from build123d import *

# Parameters (mm, degrees)
BOSS_EXTRU_1_DEPTH = 5
BOSS_EXTRU_2_DEPTH = 5


with BuildPart() as part:
    # Esquisse1 → Boss.-Extru.1 (new body)
    with BuildSketch(Plane(origin=(0, 0, 0), x_dir=(1, 0, 0), z_dir=(0, 1, 0))):
        with BuildLine():
            Line((-45.607160176, -54.708924596), (-20.666600132, -11.510607431))
            Line((-20.666600132, -11.510607431), (-20.260750016, -11.207654407))
            Line((-20.260750016, -11.207654407), (-0.260750016, -11.207654407))
            Line((-0.260750016, -11.207654407), (19.739249984, -11.207654407))
            Line((19.739249984, -11.207654407), (20.085660146, -11.407654407))
            Line((20.085660146, -11.407654407), (45.085660146, -54.708924596))
            Line((45.085660146, -54.708924596), (45.085660146, 5.291075404))
            ThreePointArc((45.085660146, 5.291075404), (-1.258158233, 50.543971712), (-45.394459717, 3.135522912))
            Line((-45.394459717, 3.135522912), (-45.607160176, -54.708924596))
        make_face()
    extrude(amount=BOSS_EXTRU_1_DEPTH)

    # Esquisse3 → Boss.-Extru.2 (add)
    with BuildSketch(Plane.XZ):
        with BuildLine():
            Line((-17.273069059, 14.232839193), (-17.133250941, 13.990667109))
            Line((-17.133250941, 13.990667109), (-16.960798401, 13.691970548))
            ThreePointArc((-16.960798401, 13.691970548), (-16.911924508, 13.553212004), (-16.916519184, 13.406169561))
            Line((-16.916519184, 13.406169561), (-16.926742719, 13.359617338))
            ThreePointArc((-16.926742719, 13.359617338), (-16.954040192, 13.27824679), (-16.998068041, 13.204572733))
            Line((-16.998068041, 13.204572733), (-17.161029392, 12.988484086))
            ThreePointArc((-17.161029392, 12.988484086), (-17.215401514, 12.92969778), (-17.280393449, 12.882919517))
            Line((-17.280393449, 12.882919517), (-25.076017394, 8.382113933))
            ThreePointArc((-25.076017394, 8.382113933), (-25.541793777, 7.256712395), (-24.574863823, 6.516089195))
            Line((-24.574863823, 6.516089195), (23.930288039, 6.572043384))
            ThreePointArc((23.930288039, 6.572043384), (24.895209417, 7.313780849), (24.429134468, 8.438068122))
            Line((24.429134468, 8.438068122), (16.801950366, 12.841624917))
            ThreePointArc((16.801950366, 12.841624917), (16.690408296, 12.921554834), (16.596603028, 13.021709699))
            Line((16.596603028, 13.021709699), (16.578320724, 13.045535661))
            ThreePointArc((16.578320724, 13.045535661), (16.457519984, 13.29049533), (16.43965666, 13.563036996))
            Line((16.43965666, 13.563036996), (16.459154582, 13.711138423))
            ThreePointArc((16.459154582, 13.711138423), (16.463606056, 13.73022975), (16.471696528, 13.748085804))
            Line((16.471696528, 13.748085804), (16.751805291, 14.233248413))
            ThreePointArc((16.751805291, 14.233248413), (16.763223851, 14.249182995), (16.777531689, 14.262583747))
            Line((16.777531689, 14.262583747), (17.093212954, 14.504814501))
            ThreePointArc((17.093212954, 14.504814501), (17.128207192, 14.52207175), (17.167141716, 14.524623654))
            Line((17.167141716, 14.524623654), (17.553917324, 14.473703679))
            ThreePointArc((17.553917324, 14.473703679), (17.57989783, 14.466626641), (17.603048157, 14.452874058))
            Line((17.603048157, 14.452874058), (17.97191114, 14.159990026))
            ThreePointArc((17.97191114, 14.159990026), (18.094102127, 14.158310543), (18.126681115, 14.276090284))
            Line((18.126681115, 14.276090284), (17.433945609, 15.973517991))
            ThreePointArc((17.433945609, 15.973517991), (17.416714959, 16.001470658), (17.391359086, 16.02233514))
            Line((17.391359086, 16.02233514), (16.076159754, 16.781665828))
            ThreePointArc((16.076159754, 16.781665828), (16.045420057, 16.793190963), (16.012604566, 16.794140313))
            Line((16.012604566, 16.794140313), (14.195418018, 16.545522578))
            ThreePointArc((14.195418018, 16.545522578), (14.109691574, 16.458410399), (14.172267612, 16.353425666))
            Line((14.172267612, 16.353425666), (14.611112944, 16.18025755))
            ThreePointArc((14.611112944, 16.18025755), (14.63461266, 16.167083269), (14.653742684, 16.148113806))
            Line((14.653742684, 16.148113806), (14.891219551, 15.838627928))
            ThreePointArc((14.891219551, 15.838627928), (14.908476799, 15.80363369), (14.911028703, 15.764699166))
            Line((14.911028703, 15.764699166), (14.859091349, 15.370195794))
            ThreePointArc((14.859091349, 15.370195794), (14.854639876, 15.351104467), (14.846549403, 15.333248413))
            Line((14.846549403, 15.333248413), (14.56644064, 14.848085804))
            ThreePointArc((14.56644064, 14.848085804), (14.55502208, 14.832151222), (14.540714242, 14.81875047))
            Line((14.540714242, 14.81875047), (14.219073364, 14.571946743))
            ThreePointArc((14.219073364, 14.571946743), (14.190371735, 14.556599446), (14.158261785, 14.551282098))
            Line((14.158261785, 14.551282098), (-0.260750016, 14.541972588))
            Line((-0.260750016, 14.541972588), (-14.596285983, 14.541972588))
            ThreePointArc((-14.596285983, 14.541972588), (-14.667470827, 14.548357651), (-14.736383073, 14.567308998))
            Line((-14.736383073, 14.567308998), (-14.843485058, 14.607357396))
            ThreePointArc((-14.843485058, 14.607357396), (-14.96184332, 14.676732873), (-15.04979813, 14.782020985))
            Line((-15.04979813, 14.782020985), (-15.227995052, 15.090667109))
            Line((-15.227995052, 15.090667109), (-15.367372917, 15.332076652))
            ThreePointArc((-15.367372917, 15.332076652), (-15.375872662, 15.351164592), (-15.380220287, 15.371602138))
            Line((-15.380220287, 15.371602138), (-15.423614857, 15.783610378))
            ThreePointArc((-15.423614857, 15.783610378), (-15.420323499, 15.821535446), (-15.403097384, 15.855482533))
            Line((-15.403097384, 15.855482533), (-15.175198809, 16.148467569))
            ThreePointArc((-15.175198809, 16.148467569), (-15.156172757, 16.167140053), (-15.132889445, 16.180122335))
            Line((-15.132889445, 16.180122335), (-14.693034359, 16.353238171))
            ThreePointArc((-14.693034359, 16.353238171), (-14.630388491, 16.458360263), (-14.716399441, 16.54540781))
            Line((-14.716399441, 16.54540781), (-16.527659803, 16.78768329))
            ThreePointArc((-16.527659803, 16.78768329), (-16.561160911, 16.786495707), (-16.59238723, 16.774303432))
            Line((-16.59238723, 16.774303432), (-17.948561264, 15.96017176))
            ThreePointArc((-17.948561264, 15.96017176), (-17.973134754, 15.939376465), (-17.98982791, 15.911851216))
            Line((-17.98982791, 15.911851216), (-18.650555766, 14.274264265))
            ThreePointArc((-18.650555766, 14.274264265), (-18.617642424, 14.156714797), (-18.495586228, 14.158572299))
            Line((-18.495586228, 14.158572299), (-18.125279987, 14.452988106))
            ThreePointArc((-18.125279987, 14.452988106), (-18.101637875, 14.466966469), (-18.075084648, 14.473985744))
            Line((-18.075084648, 14.473985744), (-17.688740592, 14.520834995))
            ThreePointArc((-17.688740592, 14.520834995), (-17.650765358, 14.518139993), (-17.616549402, 14.501447188))
            Line((-17.616549402, 14.501447188), (-17.299518527, 14.262724159))
            ThreePointArc((-17.299518527, 14.262724159), (-17.284787821, 14.249114525), (-17.273069059, 14.232839193))
        make_face()
    extrude(amount=BOSS_EXTRU_2_DEPTH)


solid = part.part
The listing builds one solid part. Answer for the finished solid, in the listing's coordinates (mm). A direction names the side the tool comes from. Round coordinates to 2 decimals unless told otherwise and drop trailing zeros. Loops run counter-clockwise (first coordinate to the right, second up) from the corner with the lowest first, then second, coordinate; pieces in that order, holes last. Notation, with made-up numbers: M 48,78.25 L 86,78.25 A13 cw 86,86.25 Z; hole C -0.5,-20 d6. An arc over 180 degrees is marked long. Write each question's results on one line, items separated by ' | '. Start each with the question number.
1) Determine the mould class of faces 6 (the flat face through (-1, 2, 11.208)), 7 (the flat face through (-21.124, -2.465, 10.664)), 8 (the flat face through (-1, -5, 11)) for opening direction Z: pulls with the +Z half, pulls with the -Z half, needs draft (parallel to the pull), parting line crosses it, or undercut.
2) Straight lines are drawn through the part: probe 1 along Y at (x, z) = (40.5, 4.5); probe 2 along Z at (x, y) = (-1, -2); probe 3 along X at (y, z) = (3, 26.5). For each, find the intervals that lie inside material, in ascending order.
3) Which of the six approach directions +Z, -Z, +X, -X, +Y, -Y give full straight-line access (tool end or side, diameter ignored) to faces 1 (the flat face through (-1, 5, -10)), 2 (the flat face through (45.086, 2, 25)), 3 (the flat face through (-1, 0, 13)), 4 (the flat face through (-33.31, 2.46, 33.41)), 5 (the flat face through (20.67, -2.46, 10.61))?
4) Find section D-D on z = 26. Write down the section's boundary in (x, y), plus the area to 3 significant figures.
5) Find section B-B on z = 40. Write down the section's boundary in (x, y).
6) Find section A-A on y = 2.75. Write down the section's boundary in (x, z), plus the area to 3 significant figures.
7) Find section C-C on x = 8.5. Write down the section's boundary in (y, z), plus the area to 3 significant figures.
8) Each of these flat-tipped pins is pushed along its axis until it touches: pin 1 (12 mm diameter, centred on x = -23, z = 38.5, fed in from +Y); pin 2 (5.5 mm diameter, centred on x = -4, y = 1.5, fed in from +Z); pin 3 (1.7 mm diameter, centred on x = -2, z = 13.5, fed in from +Y); pin 4 (6 mm diameter, centred on x = 22.5, y = -0.5, fed in from -Z). Where does it stop, or does it pass through?
Final values:
1) face 6: pulls with the +Z half | face 7: undercut | face 8: needs draft
2) probe 1: 0 to 5 | probe 2: 6.54 to 14.54 | probe 3: -45.5 to -29.32, 28.8 to 45.09
3) face 1: +Z, -Z, +X, -X, +Y | face 2: +Z, -Z, +X, +Y, -Y | face 3: +Z, +Y | face 4: +Z, +Y, -Y | face 5: +X, -Y
4) outline: M -45.5,0 L -29.03,0 L -29.03,5 L -45.5,5 Z; M 28.51,0 L 45.09,0 L 45.09,5 L 28.51,5 Z | area: 165 mm²
5) outline: M -45.55,0 L -37.11,0 L -37.11,5 L -45.55,5 Z; M 36.59,0 L 45.09,0 L 45.09,5 L 36.59,5 Z
6) outline: M -45.61,54.71 L -45.39,-3.14 A45.27 ccw long 45.09,-5.29 L 45.09,54.71 L 20.09,11.41 L 19.74,11.21 L -20.26,11.21 L -20.67,11.51 Z | area: 5,800 mm²
7) outline: M -5,6.55 L 0,6.55 L 0,-49.72 L 5,-49.72 L 5,11.21 L 0,11.21 L 0,14.55 L -5,14.55 Z | area: 345 mm²
8) pin 1: through | pin 2: z = 14.54 | pin 3: y = 0 | pin 4: z = -46.03
